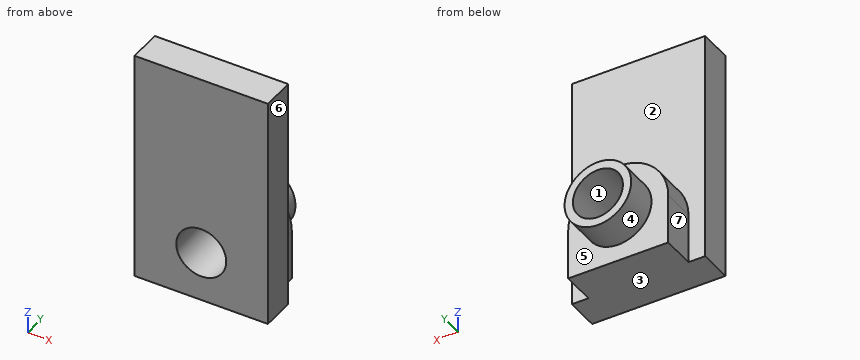
Autodesk Inventor part; units mm, degrees
ref_plane "YZ Plane" through (0, 0, 0) normal (1, 0, 0) x (0, 1, 0)
ref_plane "XZ Plane" through (0, 0, 0) normal (0, 1, 0) x (-1, 0, 0)
ref_plane "XY Plane" through (0, 0, 0) normal (0, 0, 1) x (1, 0, 0)
sketch "Sketch1" plane through (0, 0, 0) normal (0, 1, 0) x (-1, 0, 0)
  line L0 (0, 0) -> (-50.8, 0)
  line L1 (-50.8, 0) -> (-50.8, -88.9)
  line L2 (-50.8, -88.9) -> (0, -88.9)
  line L3 (0, -88.9) -> (0, 0)
  dimension "d0" = 50.8
  dimension "d1" = 88.9
extrude "Extrusion1" add sketch "Sketch1" along normal blind 12.7
sketch "Sketch2" plane through (0, 12.7, 0) normal (0, 1, 0) x (1, 0, 0)
  line L0 (50.8, 0) -> (50.8, 88.9)
  line L1 (50.8, 88.9) -> (0, 88.9)
  line L2 (0, 88.9) -> (0, 0)
  line L3 (6.35, 88.9) -> (44.45, 88.9)
  line L4 (44.45, 88.9) -> (44.45, 69.85)
  line L5 (44.45, 69.85) -> (6.35, 69.85)
  line L6 (6.35, 69.85) -> (6.35, 88.9)
  line L7 (6.35, 79.375) -> (0, 79.375) construction
  line L8 (44.45, 79.375) -> (50.8, 79.375) construction
  circle A0 centre (25.4, 69.85) radius 19.05
  dimension "d4" = 19.05
  dimension "d5" = 6.35
extrude "Extrusion2" add sketch "Sketch2" along normal blind 12.7
sketch "Sketch3" plane through (0, 25.4, 0) normal (0, 1, 0) x (1, 0, 0)
  arc A0 (6.35, 69.85) -> (44.45, 69.85) centre (25.4, 69.85) ccw
  circle A1 centre (25.4, 69.85) radius 12.7
  point P0 (0, 0)
  dimension "d8" = 25.4
extrude "Extrusion3" add sketch "Sketch3" along normal blind 12.7
sketch "Sketch6" plane through (0, 12.7, 0) normal (0, 1, 0) x (1, 0, 0)
  line L0 (44.45, 88.9) -> (44.45, 69.85)
  arc A0 (6.35, 69.85) -> (44.45, 69.85) centre (25.4, 69.85) ccw
  line L1 (6.35, 69.85) -> (6.35, 88.9)
  line L2 (6.35, 88.9) -> (0, 88.9)
  line L3 (0, 88.9) -> (0, 0)
  line L4 (0, 0) -> (50.8, 0)
  line L5 (50.8, 0) -> (50.8, 88.9)
  line L6 (50.8, 88.9) -> (44.45, 88.9)
  line L7 (44.45, 88.9) -> (44.45, 6.35) construction
  line L8 (44.45, 6.35) -> (6.35, 6.35) construction
  line L9 (6.35, 6.35) -> (6.35, 88.9) construction
  line L10 (6.35, 38.1) -> (44.45, 38.1) construction
  dimension "d35" = 6.35
  dimension "d36" = 31.75
hole "Hole3" at (25.4, 38.1, -69.85) direction (0, -1, 0) diameter 19.05 end through all
properties part number "Holes"
CAD build for the part. Positions are in the model's coordinates, mm. Face numbers are marked on the shaded views. A direction names the side the tool comes from. Round coordinates to 2 decimals unless told otherwise and drop trailing zeros. Write each loop counter-clockwise with the first axis right and the second up, starting at its lowest first coordinate (ties: lowest second). Pieces come first, ordered by that corner, then holes. Notation, with made-up numbers: M 54.25,-9.5 L 63.25,-9.5 A9 ccw 63.25,3.5 Z; hole C 19.25,19.25 d8. An arc over 180 degrees is marked long. Use a Markdown table: item, result. Add a question column.
1. 3-axis set-ups, long thin cutter, end or side, ignore diameter. For the marked faces 5, 6 and 7: which of +Z, -Z, +X, -X, +Y, -Y reach the whole face in a straight line?
2. Pull direction Z, two halves, no side cores. Call the marked faces 1, 2, 3 and 4: released by +Z, released by -Z, zero draft, split by the parting line, or undercut.
3. Flat gauge pins, fed straight in: P1, Ø10, axis at x = 30.5, y = 32.5, coming from the +Z side; P2, Ø1.5, axis at x = 16.5, y = 23.5, coming from the +Z side; P3, Ø4, axis at x = 14, z = -55, coming from the +Y side; P4, Ø17, axis at x = 25.4, z = -69.85, coming from the +Y side. Where does each tip first touch, or does it go through?
4. Slice it at C-C on z = -75. Give the cut face in (x, y), then the cut area to 3 significant figures.
5. Slice it at B-B on y = 8. Give the cut face in (x, z) (3 decimals), then the cut area to 3 significant figures.
6. Slice it at D-D on x = 31. Give the cut face in (y, z).
7. Slice it at A-A on x = 25.4. Give the cut face in (y, z) (3 decimals), then the cut area to 3 significant figures.
8. Drill centre lines: probe 1 along Z at (x, y) = (25.4, 11) (3 decimals); probe 2 along X at (y, z) = (8, -69.85) (3 decimals); probe 3 along Z at (x, y) = (25, 27). Where is each one in solid material? Low to high.
Reply:
| question | item | result |
|---|---|---|
| 1 | face 5 | +Y |
| 1 | face 6 | +Z, -Z, +X, +Y, -Y |
| 1 | face 7 | +Z, -Z, -X, +Y |
| 2 | face 1 | undercut |
| 2 | face 2 | zero draft |
| 2 | face 3 | released by -Z |
| 2 | face 4 | split by the parting line |
| 3 | P1 | stops at z = -57.15 |
| 3 | P2 | stops at z = -52.63 |
| 3 | P3 | stops at y = 25.4 |
| 3 | P4 | passes through |
| 4 | outline | M 0,0 L 17.39,0 L 17.39,38.1 L 13.79,38.1 L 13.79,25.4 L 6.35,25.4 L 6.35,12.7 L 0,12.7 Z; M 33.41,0 L 50.8,0 L 50.8,12.7 L 44.45,12.7 L 44.45,25.4 L 37.01,25.4 L 37.01,38.1 L 33.41,38.1 Z |
| 4 | area | 813 mm^2 |
| 5 | outline | M 0,-88.9 L 50.8,-88.9 L 50.8,0 L 0,0 Z; hole C 25.4,-69.85 d19.05 |
| 5 | area | 4,230 mm^2 |
| 6 | outline | M 0,-88.9 L 25.4,-88.9 L 25.4,-81.25 L 38.1,-81.25 L 38.1,-77.55 L 0,-77.55 Z; M 0,-62.15 L 38.1,-62.15 L 38.1,-58.45 L 25.4,-58.45 L 25.4,-51.64 L 12.7,-51.64 L 12.7,0 L 0,0 Z |
| 7 | outline | M 0,-88.9 L 25.4,-88.9 L 25.4,-82.55 L 38.1,-82.55 L 38.1,-79.375 L 0,-79.375 Z; M 0,-60.325 L 38.1,-60.325 L 38.1,-57.15 L 25.4,-57.15 L 25.4,-50.8 L 12.7,-50.8 L 12.7,0 L 0,0 Z |
| 7 | area | 1,210 mm^2 |
| 8 | probe 1 | z = -88.9 to -79.375, -60.325 to 0 |
| 8 | probe 2 | x = 0 to 15.875, 34.925 to 50.8 |
| 8 | probe 3 | z = -82.54 to -79.37, -60.33 to -57.16 |
